from build123d import *

# Parameters (mm, degrees)
F0_R     = 1.25
F1_DEPTH = 50
F2_R     = 5


with BuildPart() as f1:
    # F0 (on Top) → F1 (new body)
    with BuildSketch(Plane.XY):
        Polygon((10, 40), (0, 40), (0, 0), (40, 0), (40, 10), (10, 10), align=None)
        with Locations((5, 5)):
            Circle(F0_R, mode=Mode.SUBTRACT)
        with Locations((36, 5)):
            Circle(F0_R, mode=Mode.SUBTRACT)
        with Locations((5, 36)):
            Circle(F0_R, mode=Mode.SUBTRACT)
    extrude(amount=F1_DEPTH)

    # F2
    f2_edges = [f1.edges().sort_by_distance(p)[0] for p in [
        (10, 10, 25),
    ]]
    fillet(f2_edges, radius=F2_R)


solid = f1.part
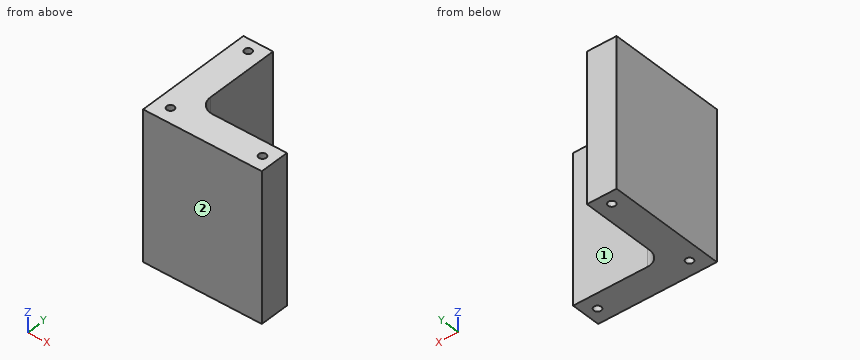
The model under review builds one solid part; all positions refer to its coordinate system, in mm. Face numbers are marked on the shaded views. A direction names the side the tool comes from. Round coordinates to 2 decimals unless told otherwise and drop trailing zeros. Loops run counter-clockwise (first coordinate to the right, second up) from the corner with the lowest first, then second, coordinate; pieces in that order, holes last. Notation, with made-up numbers: M 67.5,-25 L 106.5,-25 A16 ccw 106.5,-7 Z; hole C -32,66 d2. An arc over 180 degrees is marked long. Answer as a JSON object with one key per item and string values.
Item 1: We need section C-C, the plane y = 36. State the section outline as (x, z) points, and give its area (3 significant figures).
Check sheet entries:
{"outline": "M 0,0 L 3.75,0 L 3.75,50 L 0,50 Z; M 6.25,0 L 10,0 L 10,50 L 6.25,50 Z", "area": "375 mm2"}
Item 2: We need section A-A, the plane x = 5. State the section outline as (y, z) points.
Check sheet entries:
{"outline": "M 0,0 L 3.75,0 L 3.75,50 L 0,50 Z; M 6.25,0 L 34.75,0 L 34.75,50 L 6.25,50 Z; M 37.25,0 L 40,0 L 40,50 L 37.25,50 Z"}
Item 3: Tool access review of the marked faces 1 and 2: name each direction out of +Z, -Z, +X, -X, +Y, -Y from which nothing blocks a thin tool from reaching the whole face with its end or side.
Check sheet entries:
{"face 1": "+Z, -Z, +X, +Y", "face 2": "+Z, -Z, +X, -X, -Y"}
Item 4: We need section B-B, the plane z = 5.5. State the section outline as (x, y) points, and give its area (3 significant figures).
Check sheet entries:
{"outline": "M 0,0 L 40,0 L 40,10 L 15,10 A5 cw 10,15 L 10,40 L 0,40 Z; hole C 5,5 d2.5; hole C 5,36 d2.5; hole C 36,5 d2.5", "area": "691 mm2"}
Item 5: Clearance check with flat-ended pins moving along their axes: P1, Ø7.5, axis at y = 30, z = 23.5, coming from the +X side; P2, Ø20, axis at x = 25, z = 16.5, coming from the +Y side; P3, Ø2, axis at y = 15, z = 13.5, coming from the +X side; P4, Ø2, axis at x = 5, y = 5, coming from the -Z side. State where each tip first meets the part, or that it passes through.
Check sheet entries:
{"P1": "x = 10", "P2": "y = 10", "P3": "x = 10.1", "P4": "through"}
Item 6: For line 1 along Y through (x, z) = (5, 30.5); line 2 along X through (y, z) = (23, 12), list the stretches that pass through material, from the lowest coordinate up.
Check sheet entries:
{"line 1": "0 to 3.75, 6.25 to 34.75, 37.25 to 40", "line 2": "0 to 10"}
